```python
from build123d import *

# Parameters (mm, degrees)
IZIM2_W                     = 200
IZIM2_H                     = 100
Y_KSEKLIK_EKSTR_ZYON1_DEPTH = 20
IZIM3_R                     = 7.5
IZIM3_R_2                   = 12.5
IZIM3_R_3                   = 15
IZIM3_W                     = 6.5
IZIM3_H                     = 22
KES_EKSTR_ZYON11_DEPTH      = 12
Y_KSEKLIK_EKSTR_ZYON2_DEPTH = 6
Y_KSEKLIK_EKSTR_ZYON3_DEPTH = 50
IZIM9_W                     = 90
IZIM9_H                     = 35
KES_EKSTR_ZYON12_DEPTH      = 7
IZIM12_R                    = 1.5
KES_EKSTR_ZYON14_DEPTH      = 34.138350552
IZIM15_W                    = 196
IZIM15_H                    = 11
KES_EKSTR_ZYON15_DEPTH      = 92
IZIM16_R                    = 1.5
KES_EKSTR_ZYON16_DEPTH      = 10


with BuildPart() as part:
    # Çizim2 → Yükseklik-Ekstrüzyon1 (new body)
    with BuildSketch(Plane(origin=(0, 0, 0), x_dir=(1, 0, 0), z_dir=(0, 1, 0))):
        with Locations((-100, 50)):
            Rectangle(IZIM2_W, IZIM2_H)
    extrude(amount=Y_KSEKLIK_EKSTR_ZYON1_DEPTH)

    # Çizim3 → Kes-Ekstrüzyon11 (cut)
    with BuildSketch(Plane(origin=(0, 20, 0), x_dir=(1, 0, 0), z_dir=(0, 1, 0))):
        with Locations((-15, 15)):
            Circle(IZIM3_R)
        with Locations((-35, 15)):
            Circle(IZIM3_R)
        with Locations((-55, 15)):
            Circle(IZIM3_R)
        with Locations((-75, 15)):
            Circle(IZIM3_R)
        with Locations((-105, 17)):
            Circle(IZIM3_R_2)
        with Locations((-181, 19)):
            Circle(IZIM3_R_3)
        with Locations((-147.75, 14)):
            Rectangle(IZIM3_W, IZIM3_H)
        with Locations((-131.25, 14)):
            Rectangle(IZIM3_W, IZIM3_H)
        with BuildLine():
            ThreePointArc((-44.897916667, 68.252979968), (-40.606601718, 59.393398282), (-31.747020032, 55.102083333))
            ThreePointArc((-31.747020032, 55.102083333), (-30, 53.25), (-28.252979968, 55.102083333))
            ThreePointArc((-28.252979968, 55.102083333), (-19.393398282, 59.393398282), (-15.102083333, 68.252979968))
            ThreePointArc((-15.102083333, 68.252979968), (-13.25, 70), (-15.102083333, 71.747020032))
            ThreePointArc((-15.102083333, 71.747020032), (-19.393398282, 80.606601718), (-28.252979968, 84.897916667))
            ThreePointArc((-28.252979968, 84.897916667), (-30, 86.75), (-31.747020032, 84.897916667))
            ThreePointArc((-31.747020032, 84.897916667), (-40.606601718, 80.606601718), (-44.897916667, 71.747020032))
            ThreePointArc((-44.897916667, 71.747020032), (-46.75, 70), (-44.897916667, 68.252979968))
        make_face()
    extrude(amount=-KES_EKSTR_ZYON11_DEPTH, mode=Mode.SUBTRACT)

    # Çizim7 → Yükseklik-Ekstrüzyon2 (add)
    with BuildSketch(Plane(origin=(0, 20, 0), x_dir=(1, 0, 0), z_dir=(0, 1, 0))):
        with BuildLine():
            Line((-112.679491924, -5), (-87.320508076, -5))
            Line((-87.320508076, -5), (-73.480762114, -12.990381057))
            ThreePointArc((-73.480762114, -12.990381057), (-69.86304779, -14.488887394), (-65.980762114, -15))
            Line((-65.980762114, -15), (0.5, -15))
            ThreePointArc((0.5, -15), (6.156854249, -12.656854249), (8.5, -7))
            Line((8.5, -7), (8.5, 97))
            ThreePointArc((8.5, 97), (-2.629942315, 123.870057685), (-29.5, 135))
            Line((-29.5, 135), (-170.5, 135))
            ThreePointArc((-170.5, 135), (-197.370057685, 123.870057685), (-208.5, 97))
            Line((-208.5, 97), (-208.5, -7))
            ThreePointArc((-208.5, -7), (-206.156854249, -12.656854249), (-200.5, -15))
            Line((-200.5, -15), (-134.019237886, -15))
            ThreePointArc((-134.019237886, -15), (-130.13695221, -14.488887394), (-126.519237886, -12.990381057))
            Line((-126.519237886, -12.990381057), (-112.679491924, -5))
        make_face()
        with BuildLine():
            Line((-71.5, 0), (-128.5, 0))
            Line((-128.5, 0), (-128.5, -2.5))
            ThreePointArc((-128.5, -2.5), (-129.085786438, -3.914213562), (-130.5, -4.5))
            Line((-130.5, -4.5), (-186.5, -4.5))
            ThreePointArc((-186.5, -4.5), (-187.914213562, -3.914213562), (-188.5, -2.5))
            Line((-188.5, -2.5), (-188.5, 0))
            Line((-188.5, 0), (-200, 0))
            Line((-200, 0), (-200, 100))
            Line((-200, 100), (0, 100))
            Line((0, 100), (0, 0))
            Line((0, 0), (-11.5, 0))
            Line((-11.5, 0), (-11.5, -2.5))
            ThreePointArc((-11.5, -2.5), (-12.085786438, -3.914213562), (-13.5, -4.5))
            Line((-13.5, -4.5), (-69.5, -4.5))
            ThreePointArc((-69.5, -4.5), (-70.914213562, -3.914213562), (-71.5, -2.5))
            Line((-71.5, -2.5), (-71.5, 0))
        make_face(mode=Mode.SUBTRACT)
    extrude(amount=-Y_KSEKLIK_EKSTR_ZYON2_DEPTH)

    # Çizim8 → Yükseklik-Ekstrüzyon3 (add, symmetric)
    with BuildSketch(Plane(origin=(-100, 0, 0), x_dir=(0, 0, -1), z_dir=(1, 0, 0))):
        Polygon((85, 20), (125.311288741, 40), (125.311288741, 20), align=None)
    extrude(amount=Y_KSEKLIK_EKSTR_ZYON3_DEPTH, both=True)

    # Çizim9 → Kes-Ekstrüzyon12 (cut)
    with BuildSketch(Plane(origin=(0, -17.792193018, -8.827399755), x_dir=(1, 0, 0), z_dir=(0, 0.895806416, 0.444444444))):
        with Locations((-100, 107.532434289)):
            Rectangle(IZIM9_W, IZIM9_H)
    extrude(amount=-KES_EKSTR_ZYON12_DEPTH, mode=Mode.SUBTRACT)

    # Çizim12 → Kes-Ekstrüzyon14 (cut, through all)
    with BuildSketch(Plane(origin=(0, -24.062837933, -11.938510866), x_dir=(1, 0, 0), z_dir=(0, 0.895806416, 0.444444444))):
        with Locations((-140, 119.032434289)):
            Circle(IZIM12_R)
        with Locations((-60, 119.032434289)):
            Circle(IZIM12_R)
    extrude(amount=-KES_EKSTR_ZYON14_DEPTH, mode=Mode.SUBTRACT)

    # Çizim15 → Kes-Ekstrüzyon15 (cut)
    with BuildSketch(Plane(origin=(0, 0, -95), x_dir=(-1, 0, 0), z_dir=(0, 0, -1))):
        with Locations((100, 7)):
            Rectangle(IZIM15_W, IZIM15_H)
    extrude(amount=-KES_EKSTR_ZYON15_DEPTH, mode=Mode.SUBTRACT)

    # Çizim16 → Kes-Ekstrüzyon16 (cut)
    with BuildSketch(Plane(origin=(0, 0, -100), x_dir=(-1, 0, 0), z_dir=(0, 0, -1))):
        with Locations((65, 8)):
            Circle(IZIM16_R)
        with Locations((135, 8)):
            Circle(IZIM16_R)
    extrude(amount=-KES_EKSTR_ZYON16_DEPTH, mode=Mode.SUBTRACT)


solid = part.part
```
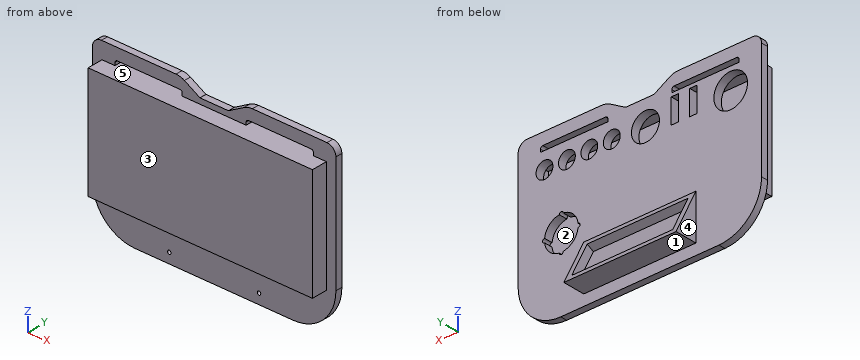
Here's how the part is built. I have some questions about the finished solid (model axes, mm). Face numbers are marked on the shaded views. A direction names the side the tool comes from. Coordinates: 2 decimals unless noted, no trailing zeros. Write each loop counter-clockwise with the first axis right and the second up, starting at its lowest first coordinate (ties: lowest second). Pieces come first, ordered by that corner, then holes. Notation, with made-up numbers: (-14, -7.75) -> (23, -7.75) arc R18 cw to (23, 5.25) -> close; hole circle Ø6 at (29, -33.5). An arc over 180 degrees is marked (long way). Use a Markdown table: item, result. Add a question column.
(1) We'd pull the mould along Y, two halves only. Please class the marked faces 1, 2 and 3: +Y half, -Y half, draft (parallel to the pull), parting line (faces both ways), or undercut.
(2) If we section it at B-B, the plane x = -180: Write out the boundary of the cut face in (y, z), and give its area (3 significant figures).
(3) If we section it at A-A, the plane x = -157.5: Write out the boundary of the cut face in (y, z), and give its area (3 significant figures).
(4) If we section it at C-C, the plane y = 35.5: Write out the boundary of the cut face in (x, z), and give its area (3 significant figures).
(5) If we section it at D-D, the plane x = -34: Write out the boundary of the cut face in (y, z).
(6) I'm going to push flat-ended pins straight in: P1, Ø4, axis at x = -126.5, y = 6.5, coming from the -Z side; P2, Ø8, axis at x = -149.5, z = -35.5, coming from the +Y side; P3, Ø8, axis at x = -116.5, z = -83, coming from the +Y side. Where does each tip first touch, or does it pass through?
(7) Please list where these lines run through material, in increasing order: line 1 (Z direction, x = -181, y = 14.75); line 2 (Z direction, x = -55, y = 14.75); line 3 (Y direction, x = -144, z = -45).
(8) For the marked faces 4 and 5, which set-ups out of +Z, -Z, +X, -X, +Y, -Y let a thin tool reach every point of the face, with its end or its side?
Outcome:
| question | item | result |
|---|---|---|
| 1 | face 1 | draft |
| 1 | face 2 | undercut |
| 1 | face 3 | -Y half |
| 2 | outline | (0, -100) -> (14, -100) -> (14, -133.79) -> (20, -133.79) -> (20, -33.97) -> (12.5, -33.97) -> (12.5, -95) -> (1.5, -95) -> (1.5, -3) -> (12.5, -3) -> (12.5, -4.03) -> (20, -4.03) -> (20, 0) -> (0, 0) -> close; (14, 4.5) -> (20, 4.5) -> (20, 15) -> (14, 15) -> close |
| 2 | area | 1,030 mm^2 |
| 3 | outline | (0, -100) -> (14, -100) -> (14, -135) -> (20, -135) -> (20, 0) -> (0, 0) -> close; (14, 4.5) -> (20, 4.5) -> (20, 15) -> (14, 15) -> close; hole (1.5, -95) -> (12.5, -95) -> (12.5, -3) -> (1.5, -3) -> close |
| 3 | area | 1,260 mm^2 |
| 4 | outline | (-150, -125.31) -> (-50, -125.31) -> (-50, -116.24) -> (-55, -116.24) -> (-55, -121.96) -> (-145, -121.96) -> (-145, -116.24) -> (-150, -116.24) -> close |
| 4 | area | 392 mm^2 |
| 5 | outline | (0, -100) -> (14, -100) -> (14, -135) -> (20, -135) -> (20, -84.46) -> (12.5, -84.46) -> (12.5, -95) -> (1.5, -95) -> (1.5, -3) -> (12.5, -3) -> (12.5, -7.57) -> (20, -7.57) -> (20, 0) -> (0, 0) -> close; (12.5, -55.54) -> (20, -55.54) -> (20, -22.43) -> (12.5, -22.43) -> close; (14, 4.5) -> (20, 4.5) -> (20, 15) -> (14, 15) -> close |
| 6 | P1 | stops at z = -100 |
| 6 | P2 | stops at y = 20 |
| 6 | P3 | stops at y = 20.99 |
| 7 | line 1 | z = -133.52 to -34, -4 to 0, 4.5 to 15 |
| 7 | line 2 | z = -135 to -22.5, -7.5 to 0, 4.5 to 15 |
| 7 | line 3 | y = 0 to 1.5, 12.5 to 20 |
| 8 | face 4 | +Z, -Z, -X, +Y |
| 8 | face 5 | -Y |
